The figure shows three views and two pictorial views of one solid part (mm, origin at its lowest corner). Answer the questions. A direction names the side the tool comes from. Round coordinates to 2 decimals unless told otherwise and drop trailing zeros. Order: outer loops, then holes, each group sorted by start corner. A loop starts at its lowest first (then second) coordinate and runs counter-clockwise, first axis right, second up. Notation, with made-up numbers: (69.5, 44.5) - (116.5, 44.5) arc R6 ccw to (116.5, 50.5) - close; hole circle Ø4 at (69, -2.75). An arc over 180 degrees is marked (long way). Answer in a Markdown table with one row per item.
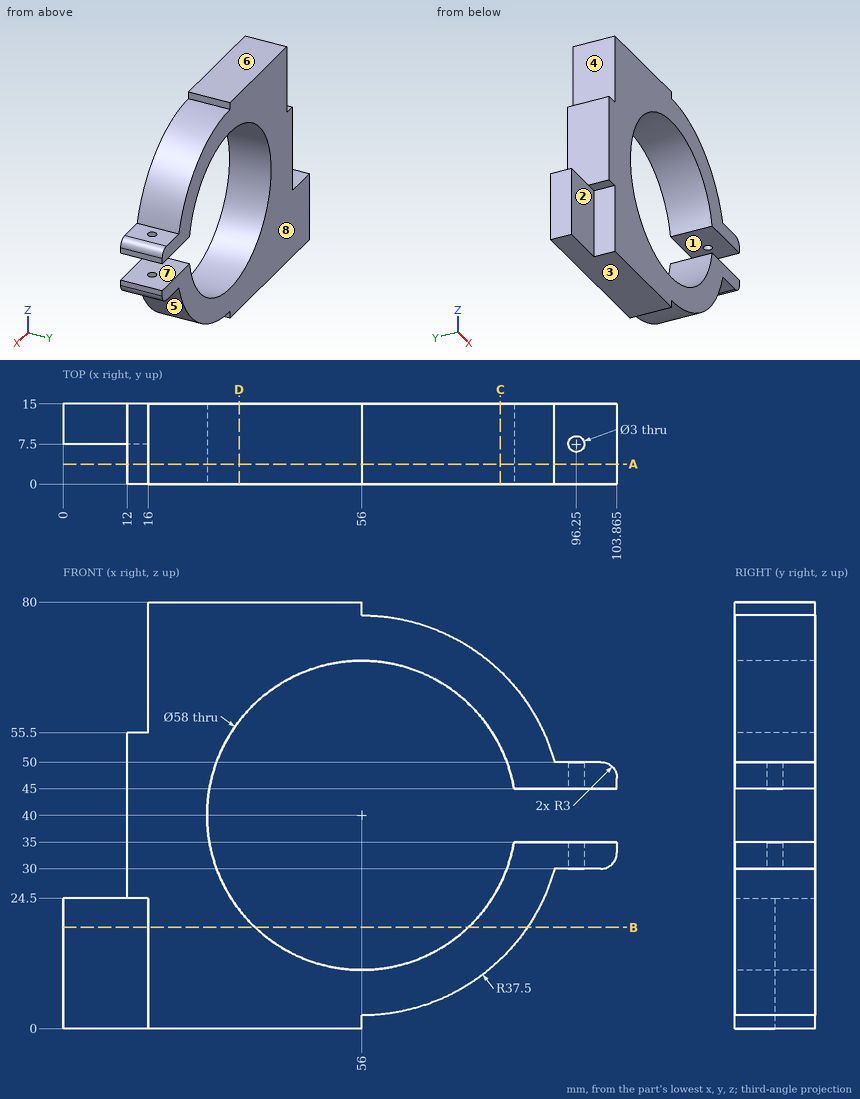
1) Find section D-D, the plane x = 33. Give the vertices of the cut face in (y, z), then the cut area to 3 significant figures.
Filled in:
| item | result |
|---|---|
| outline | (0, 0) - (15, 0) - (15, 22.34) - (0, 22.34) - close; (0, 57.66) - (15, 57.66) - (15, 80) - (0, 80) - close |
| area | 670 mm^2 |
2) Which of the six approach directions +Z, -Z, +X, -X, +Y, -Y give full straight-line access (tool end or side, diameter ignored) to the marked faces 1, 2, 3, 4 and 5?
Filled in:
| item | result |
|---|---|
| face 1 | +X, +Y, -Y |
| face 2 | -Z, -X, -Y |
| face 3 | -Z, +X, -X, +Y, -Y |
| face 4 | +Z, -X, +Y, -Y |
| face 5 | -Z, +X, +Y, -Y |
3) Find section B-B, the plane z = 19. Give the vertices of the cut face in (x, y).
Filled in:
| item | result |
|---|---|
| outline | (0, 7.5) - (16, 7.5) - (16, 0) - (36, 0) - (36, 15) - (0, 15) - close; (76, 0) - (87.07, 0) - (87.07, 15) - (76, 15) - close |
4) Find section C-C, the plane x = 82. Give the vertices of the cut face in (y, z) (1 decimal), then the cut area to 3 significant figures.
Filled in:
| item | result |
|---|---|
| outline | (0, 13) - (15, 13) - (15, 27.2) - (0, 27.2) - close; (0, 52.8) - (15, 52.8) - (15, 67) - (0, 67) - close |
| area | 425 mm^2 |
5) Each of these flat-tipped pins is pushed along its axis until it touches: pin 1 (2 mm diameter, centred on x = 4.5, y = 10, fed in from +Z); pin 2 (2 mm diameter, centred on x = 68.5, y = 1.5, fed in from +Z); pin 3 (7.5 mm diameter, centred on x = 97.5, y = 8.5, fed in from +Z); pin 4 (2.5 mm diameter, centred on x = 96.25, y = 7.5, fed in from -Z). Where does it stop, or does it pass through?
Filled in:
| item | result |
|---|---|
| pin 1 | stops at z = 24.5 |
| pin 2 | stops at z = 75.69 |
| pin 3 | stops at z = 50 |
| pin 4 | passes through |
6) Find section A-A, the plane y = 3.75. Give the vertices of the cut face in (x, z) (1 decimal).
Filled in:
| item | result |
|---|---|
| outline | (12, 24.5) - (16, 24.5) - (16, 0) - (56, 0) - (56, 2.5) arc R37.5 ccw to (92.1, 30) - (100.9, 30) arc R3 ccw to (103.9, 33) - (103.9, 35) - (84.6, 35) arc R29 cw (long way) to (84.6, 45) - (103.9, 45) - (103.9, 47) arc R3 ccw to (100.9, 50) - (92.1, 50) arc R37.5 ccw to (56, 77.5) - (56, 80) - (16, 80) - (16, 55.5) - (12, 55.5) - close |
7) The mould has two halves that part along Z. Classify the marked faces 6, 7 and 8: released by +Z, released by -Z, zero draft, split by the parting line, or undercut.
Filled in:
| item | result |
|---|---|
| face 6 | released by +Z |
| face 7 | undercut |
| face 8 | zero draft |
8) Find the intervals of material crossed by probe 1 along Z at (x, y) = (99, 1); probe 2 along X at (y, z) = (7.5, 47.95); probe 3 along X at (y, z) = (6.25, 25.5) (1 decimal), in increasing order. Write a range as from..to.
Filled in:
| item | result |
|---|---|
| probe 1 | z = 30..35, 45..50 |
| probe 2 | x = 12..28.11, 83.89..94.75, 97.75..103.71 |
| probe 3 | x = 12..30.9, 81.1..90.6 |
